Here's the drawing with two shaded views (mm, measured from the low corner). I have some questions. Coordinates: 2 decimals unless noted, no trailing zeros. Write each loop counter-clockwise with the first axis right and the second up, starting at its lowest first coordinate (ties: lowest second). Pieces come first, ordered by that corner, then holes. Notation, with made-up numbers: (69.25, -34.5) -> (80.25, -34.5) arc R16 cw to (80.25, -13.5) -> close; hole circle Ø11 at (-22, -23). An arc over 180 degrees is marked (long way). Use a Markdown table: item, result. Add a question column.
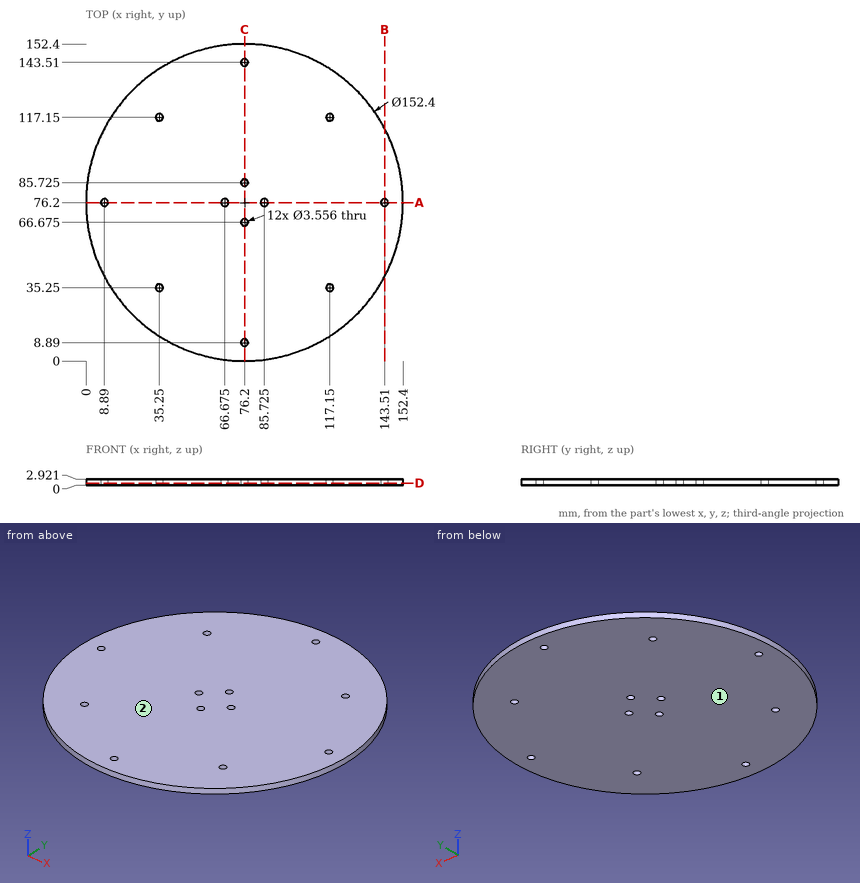
Q1. Please list where these lines run through material, in increasing order: line 1 (Y direction, x = 76.5, z = 0.6); line 2 (X direction, y = 143.51, z = 1); line 3 (X direction, y = 85, z = 1.8).
Q2. Thinking about a two-plate mould opening in Z: for the marked faces 1 and 2, which applies, released by +Z, released by -Z, zero draft, split by the parting line, or undercut?
Q3. Suppose I cut it at A-A, the plane y = 76.2. Write out the boundary of the cut face in (x, z).
Q4. Suppose I cut it at D-D, the plane z = 0.9. State how many separate pieces and enclosed holes the cut face has, and give its area (3 significant figures).
Q5. Suppose I cut it at B-B, the plane x = 143.51. Write out the boundary of the cut face in (y, z), and give its area (3 significant figures).
Q6. Will these pins go through, and if not, where does the flat tip stop? pin 1 (1.5 mm diameter, centred on x = 57.5, z = 2, fed in from +Y); pin 2 (1 mm diameter, centred on y = 15.5, z = 1, fed in from +X).
Answer key:
| question | item | result |
|---|---|---|
| 1 | line 1 | y = 0 to 7.14, 10.64 to 64.92, 68.43 to 83.97, 87.48 to 141.76, 145.26 to 152.4 |
| 1 | line 2 | x = 40.48 to 74.42, 77.98 to 111.92 |
| 1 | line 3 | x = 0.51 to 74.58, 77.82 to 151.89 |
| 2 | face 1 | released by -Z |
| 2 | face 2 | released by +Z |
| 3 | outline | (0, 0) -> (7.11, 0) -> (7.11, 2.92) -> (0, 2.92) -> close; (10.67, 0) -> (64.9, 0) -> (64.9, 2.92) -> (10.67, 2.92) -> close; (68.45, 0) -> (83.95, 0) -> (83.95, 2.92) -> (68.45, 2.92) -> close; (87.5, 0) -> (141.73, 0) -> (141.73, 2.92) -> (87.5, 2.92) -> close; (145.29, 0) -> (152.4, 0) -> (152.4, 2.92) -> (145.29, 2.92) -> close |
| 4 | separate pieces | 1 |
| 4 | enclosed holes | 12 |
| 4 | area | 18,100 mm^2 |
| 5 | outline | (40.48, 0) -> (74.42, 0) -> (74.42, 2.92) -> (40.48, 2.92) -> close; (77.98, 0) -> (111.92, 0) -> (111.92, 2.92) -> (77.98, 2.92) -> close |
| 5 | area | 198 mm^2 |
| 6 | pin 1 | stops at y = 150.26 |
| 6 | pin 2 | stops at x = 122.92 |
